Work out the finished part from the listing and answer in its coordinate system (mm). A direction names the side the tool comes from. Round coordinates to 2 decimals unless told otherwise and drop trailing zeros. Write each loop counter-clockwise with the first axis right and the second up, starting at its lowest first coordinate (ties: lowest second). Pieces come first, ordered by that corner, then holes. Notation, with made-up numbers: (4.5, 50.5) -> (23.5, 50.5) arc R27 cw to (23.5, 71.5) -> close; hole circle Ø10 at (14, -1). An arc over 180 degrees is marked (long way). One line per item, written item: value.
```python
from build123d import *

# Parameters (mm, degrees)
SKETCH1_W                = 100
SKETCH1_H                = 100
BOSS_EXTRUDE1_DEPTH      = 250
SKETCH2_W                = 90
SKETCH2_H                = 90
CUT_EXTRUDE1_DEPTH       = 288.228132327
FILLET1_R                = 10.16
SKETCH3_W                = 9.3412
SKETCH3_H                = 5
BOSS_EXTRUDE2_DEPTH      = 250
SKETCH4_W                = 100
SKETCH4_H                = 125
CUT_EXTRUDE2_DEPTH       = 288.228132327
SKETCH6_W                = 81
SKETCH6_H                = 100
CUT_EXTRUDE4_DEPTH       = 5
FILLET3_R                = 10.16
BOSS_EXTRUDE3_DEPTH      = 30.48
SKETCH9_W                = 81
SKETCH9_H                = 6.25
BOSS_EXTRUDE5_DEPTH      = 35.052
CUT_EXTRUDE5_DEPTH       = 2
SKETCH12_W               = 81
SKETCH12_H               = 2.848
CUT_EXTRUDE6_DEPTH       = 24.23
SKETCH13_W               = 2.5
SKETCH13_H               = 31.9
SKETCH13_H_2             = 27
BOSS_EXTRUDE6_DEPTH      = 40
SKETCH14_W               = 2.63
SKETCH14_H               = 32.03
SKETCH14_W_2             = 2.37
SKETCH14_H_2             = 31.77
SKETCH14_H_3             = 27.13
SKETCH14_H_4             = 26.87
CUT_EXTRUDE10_DEPTH      = 40
CUT_EXTRUDE11_DEPTH      = 6.25
CUT_EXTRUDE12_DEPTH      = 173.497863465
CUT_EXTRUDE12_DEPTH_BACK = 173.497863465
BOSS_EXTRUDE7_DEPTH      = 24.23
CUT_EXTRUDE14_REACH      = 287.489
SKETCH20_W               = 89
SKETCH20_H               = 102.5


with BuildPart() as part:
    # Sketch1 → Boss-Extrude1 (new body)
    with BuildSketch(Plane.XY):
        with Locations((50, 50)):
            Rectangle(SKETCH1_W, SKETCH1_H)
    extrude(amount=BOSS_EXTRUDE1_DEPTH)

    # Sketch2 → Cut-Extrude1 (cut, through all)
    with BuildSketch(Plane(origin=(0, 0, 0), x_dir=(-1, 0, 0), z_dir=(0, 0, -1))):
        with Locations((-50, 50)):
            Rectangle(SKETCH2_W, SKETCH2_H)
    extrude(amount=-CUT_EXTRUDE1_DEPTH, mode=Mode.SUBTRACT)

    # Fillet1
    fillet1_edges = [part.edges().sort_by_distance(p)[0] for p in [
        (0, 100, 125),
        (0, 0, 125),
        (100, 0, 125),
        (100, 100, 125),
    ]]
    fillet(fillet1_edges, radius=FILLET1_R)

    # Sketch3 → Boss-Extrude2 (add, through all)
    with BuildSketch(Plane(origin=(0, 0, 0), x_dir=(-1, 0, 0), z_dir=(0, 0, -1))):
        with Locations((-90.3294, 55.4)):
            Rectangle(SKETCH3_W, SKETCH3_H)
        with Locations((-90.3294, 44.6)):
            Rectangle(SKETCH3_W, SKETCH3_H)
        with Locations((-9.6706, 44.6)):
            Rectangle(SKETCH3_W, SKETCH3_H)
        with Locations((-9.6706, 55.4)):
            Rectangle(SKETCH3_W, SKETCH3_H)
    extrude(amount=-BOSS_EXTRUDE2_DEPTH)

    # Sketch4 → Cut-Extrude2 (cut, through all)
    with BuildSketch(Plane(origin=(0, 100, 0), x_dir=(1, 0, 0), z_dir=(0, 1, 0))):
        with Locations((50, -62.5)):
            Rectangle(SKETCH4_W, SKETCH4_H)
    extrude(amount=-CUT_EXTRUDE2_DEPTH, mode=Mode.SUBTRACT)

    # Sketch6 → Cut-Extrude4 (cut)
    with BuildSketch(Plane.XZ):
        with Locations((50, 175)):
            Rectangle(SKETCH6_W, SKETCH6_H)
    extrude(amount=-CUT_EXTRUDE4_DEPTH, mode=Mode.SUBTRACT)

    # Fillet3
    fillet3_edges = [part.edges().sort_by_distance(p)[0] for p in [
        (5, 95, 187.5),
        (5, 5, 187.5),
        (95, 95, 187.5),
        (95, 5, 187.5),
    ]]
    fillet(fillet3_edges, radius=FILLET3_R)

    # Sketch7 → Boss-Extrude3 (add)
    with BuildSketch(Plane(origin=(0, 0, 125), x_dir=(-1, 0, 0), z_dir=(0, 0, -1))):
        Polygon((-95, 96), (-5, 96), (-5, 57.9), (-9.5, 57.9), (-9.5, 92.952), (-90.5, 92.952), (-90.5, 57.9), (-95, 57.9), align=None)
    extrude(amount=-BOSS_EXTRUDE3_DEPTH)

    # Sketch9 → Boss-Extrude5 (add)
    with BuildSketch(Plane.XZ.offset(-92.952)):
        with Locations((50, 152.355)):
            Rectangle(SKETCH9_W, SKETCH9_H)
    extrude(amount=BOSS_EXTRUDE5_DEPTH)

    # Sketch10 → Cut-Extrude5 (cut)
    with BuildSketch(Plane.XY.offset(250)):
        with BuildLine():
            Line((89.84, 100), (10.16, 100))
            ThreePointArc((10.16, 100), (2.975795103, 97.024204897), (0, 89.84))
            Line((0, 89.84), (0, 10.16))
            ThreePointArc((0, 10.16), (2.975795103, 2.975795103), (10.16, 0))
            Line((10.16, 0), (89.84, 0))
            ThreePointArc((89.84, 0), (97.024204897, 2.975795103), (100, 10.16))
            Line((100, 10.16), (100, 89.84))
            ThreePointArc((100, 89.84), (97.024204897, 97.024204897), (89.84, 100))
        make_face()
    extrude(amount=-CUT_EXTRUDE5_DEPTH, mode=Mode.SUBTRACT)

    # Sketch12 → Cut-Extrude6 (cut)
    with BuildSketch(Plane(origin=(0, 0, 125), x_dir=(-1, 0, 0), z_dir=(0, 0, -1))):
        with Locations((-50, 94.376)):
            Rectangle(SKETCH12_W, SKETCH12_H)
    extrude(amount=-CUT_EXTRUDE6_DEPTH, mode=Mode.SUBTRACT)

    # Sketch13 → Boss-Extrude6 (add)
    with BuildSketch(Plane(origin=(0, 0, 125), x_dir=(-1, 0, 0), z_dir=(0, 0, -1))):
        with Locations((-97.5, 73.85)):
            Rectangle(SKETCH13_W, SKETCH13_H)
        with Locations((-97.5, 26.1)):
            Rectangle(SKETCH13_W, SKETCH13_H_2)
        with Locations((-2.5, 26.1)):
            Rectangle(SKETCH13_W, SKETCH13_H_2)
        with Locations((-2.5, 73.85)):
            Rectangle(SKETCH13_W, SKETCH13_H)
    extrude(amount=BOSS_EXTRUDE6_DEPTH)

    # Sketch14 → Cut-Extrude10 (cut)
    # profile 1 of 4: a face of its own
    with BuildSketch(Plane(origin=(0, 0, 125), x_dir=(-1, 0, 0), z_dir=(0, 0, -1))):
        with Locations((-97.5, 73.85)):
            Rectangle(SKETCH14_W, SKETCH14_H)
        with Locations((-97.5, 73.85)):
            Rectangle(SKETCH14_W_2, SKETCH14_H_2, mode=Mode.SUBTRACT)
    # profile 2 of 4: a face of its own
    with BuildSketch(Plane(origin=(0, 0, 125), x_dir=(-1, 0, 0), z_dir=(0, 0, -1))):
        with Locations((-2.5, 73.85)):
            Rectangle(SKETCH14_W, SKETCH14_H)
        with Locations((-2.5, 73.85)):
            Rectangle(SKETCH14_W_2, SKETCH14_H_2, mode=Mode.SUBTRACT)
    # profile 3 of 4: a face of its own
    with BuildSketch(Plane(origin=(0, 0, 125), x_dir=(-1, 0, 0), z_dir=(0, 0, -1))):
        with Locations((-97.5, 26.1)):
            Rectangle(SKETCH14_W, SKETCH14_H_3)
        with Locations((-97.5, 26.1)):
            Rectangle(SKETCH14_W_2, SKETCH14_H_4, mode=Mode.SUBTRACT)
    # profile 4 of 4: a face of its own
    with BuildSketch(Plane(origin=(0, 0, 125), x_dir=(-1, 0, 0), z_dir=(0, 0, -1))):
        with Locations((-2.5, 26.1)):
            Rectangle(SKETCH14_W, SKETCH14_H_3)
        with Locations((-2.5, 26.1)):
            Rectangle(SKETCH14_W_2, SKETCH14_H_4, mode=Mode.SUBTRACT)
    extrude(amount=CUT_EXTRUDE10_DEPTH, mode=Mode.SUBTRACT)

    # Sketch15 → Cut-Extrude11 (cut)
    with BuildSketch(Plane.XY.offset(155.48)):
        with BuildLine():
            Line((5, 57.9), (14.3412, 57.9))
            Line((14.3412, 57.9), (85.6588, 57.9))
            Line((85.6588, 57.9), (95, 57.9))
            Line((95, 57.9), (95, 84.84))
            ThreePointArc((95, 84.84), (92.024204897, 92.024204897), (84.84, 95))
            Line((84.84, 95), (15.16, 95))
            ThreePointArc((15.16, 95), (7.975795103, 92.024204897), (5, 84.84))
            Line((5, 84.84), (5, 57.9))
        make_face()
    extrude(amount=-CUT_EXTRUDE11_DEPTH, mode=Mode.SUBTRACT)

    # Sketch16 → Cut-Extrude12 (cut, two sides: drawn at the far end of the back side and taken through both)
    with BuildSketch(Plane.XY.offset(149.23).offset(-CUT_EXTRUDE12_DEPTH_BACK)):
        with BuildLine():
            Line((5, 57.9), (95, 57.9))
            Line((95, 57.9), (95, 84.84))
            ThreePointArc((95, 84.84), (92.024204897, 92.024204897), (84.84, 95))
            Line((84.84, 95), (15.16, 95))
            ThreePointArc((15.16, 95), (7.975795103, 92.024204897), (5, 84.84))
            Line((5, 84.84), (5, 57.9))
        make_face()
    extrude(amount=CUT_EXTRUDE12_DEPTH + CUT_EXTRUDE12_DEPTH_BACK, mode=Mode.SUBTRACT)

    # Sketch17 → Boss-Extrude7 (add)
    with BuildSketch(Plane(origin=(0, 0, 149.23), x_dir=(-1, 0, 0), z_dir=(0, 0, -1))):
        with BuildLine():
            Line((-84.84, 95), (-15.16, 95))
            ThreePointArc((-15.16, 95), (-12.201837845, 94.559818757), (-9.5, 93.277416666))
            Line((-9.5, 93.277416666), (-9.5, 95.8))
            Line((-9.5, 95.8), (-90.5, 95.8))
            Line((-90.5, 95.8), (-90.5, 93.277416666))
            ThreePointArc((-90.5, 93.277416666), (-87.798162155, 94.559818757), (-84.84, 95))
        make_face()
    extrude(amount=BOSS_EXTRUDE7_DEPTH)

    # Cut-Extrude14: up to this face of the body (flat: up to its plane)
    cut_extrude14_end = Plane(part.part.faces().sort_by_distance((9.6706, 42.1, 186.5))[0])
    # Sketch20 → Cut-Extrude14 (cut, up to the picked face)
    with BuildSketch(Plane.XZ, mode=Mode.PRIVATE) as cut_extrude14_sk1:
        with Locations((50, 176.25)):
            Rectangle(SKETCH20_W, SKETCH20_H)
    cut_extrude14_tool1 = split(extrude(cut_extrude14_sk1.sketch, amount=-CUT_EXTRUDE14_REACH, mode=Mode.PRIVATE), bisect_by=cut_extrude14_end, keep=Keep.BOTH, mode=Mode.PRIVATE)
    add(cut_extrude14_tool1.solids().sort_by(Axis((50, 0, 176.25), (0, 1, 0)))[0], mode=Mode.SUBTRACT)


solid = part.part
```
(1) Consider probe 1 along Y at (x, z) = (9.5, 167); probe 2 along X at (y, z) = (30.5, 116.5) (3 decimals); probe 3 along X at (y, z) = (14.5, 160). Determine where each line is inside the solid, lowest interval first.
Reported:
probe 1: y = 42.1 to 47.1, 52.9 to 57.9, 93.28 to 99.98
probe 2: x = 1.315 to 3.685, 96.315 to 98.685
probe 3: x = 0 to 5.02, 94.98 to 100
(2) Flat-ended cylindrical pins translate along their axes: pin 1 Ø1.2 at (x, z) = (97, 113.5) entering from +Y (3 decimals); pin 2 Ø13.5 at (y, z) = (25.5, 103.5) entering from -X (3 decimals); pin 3 Ø0.7 at (x, z) = (2.5, 103) entering from -Y (3 decimals); pin 4 Ø3 at (x, z) = (90.5, 190) entering from +Y. Find the tip coordinate at first contact, or state that the pin passes through.
Reported:
pin 1: stops at y = 89.735
pin 2: stops at x = 1.315
pin 3: stops at y = 12.665
pin 4: stops at y = 100
(3) For a pull along Y with two mould halves and no side action, classify faces 6 (the face through (10, 57.9, 186)), 7 (the face through (5, 28, 186)), 8 (the face through (49, 100, 186)), 9 (the face through (12.7, 46.5, 248)) as pulls with the +Y half, pulls with the -Y half, needs draft (parallel to the pull), parting line crosses it, or undercut.
Reported:
face 6: undercut
face 7: undercut
face 8: pulls with the +Y half
face 9: needs draft
(4) Find section C-C on x = 58.5. Give the vertices of the cut face in (y, z), plus the area to 4 significant figures.
Reported:
outline: (0, 227.5) -> (5, 227.5) -> (5, 248) -> (0, 248) -> close; (95, 125) -> (100, 125) -> (100, 248) -> (95, 248) -> close
area: 717.5 mm2
(5) Find section A-A on y = 70. Give the vertices of the cut face in (x, z) (3 decimals).
Reported:
outline: (0, 125) -> (1.315, 125) -> (1.315, 85) -> (3.685, 85) -> (3.685, 125) -> (5, 125) -> (5, 248) -> (0, 248) -> close; (95, 125) -> (96.315, 125) -> (96.315, 85) -> (98.685, 85) -> (98.685, 125) -> (100, 125) -> (100, 248) -> (95, 248) -> close
(6) A tool of negligible diameter and unlimited length cuts with its end or side. For faces 1 (the face through (1.774, 4.424, 187.361)), 2 (the face through (94.5, 6, 176)), 3 (the face through (96.315, 74, 105)), 4 (the face through (98.685, 26, 105)), 5 (the face through (90, 57.9, 186)), from which of +Z, -Z, +X, -X, +Y, -Y can it reach the whole face along a straight path? Write none if from no direction.
Reported:
face 1: +Z, -Z, -X, -Y
face 2: -Z, -Y
face 3: -Z, +Y, -Y
face 4: -Z, +X, +Y, -Y
face 5: +Z, -Z
